```python
from build123d import *

# Parameters (mm, degrees)
BOSS_EXTRUDE1_DEPTH       = 9
SKETCH2_W                 = 3
SKETCH2_H                 = 1
SKETCH2_H_2               = 7.797958972
CUT_EXTRUDE1_DEPTH        = 19
SKETCH3_R                 = 4.5
BOSS_EXTRUDE2_DEPTH       = 6
SKETCH4_R                 = 3
BOSS_EXTRUDE3_DEPTH       = 3
F_3_0MM_DOWEL_HOLE1_D     = 3
F_3_0MM_DOWEL_HOLE1_DEPTH = 4
F_3_0MM_DOWEL_HOLE1_TIP   = 0.901290929
CUT_EXTRUDE2_DEPTH        = 3


with BuildPart() as part:
    # Sketch1 → Boss-Extrude1 (new body)
    with BuildSketch(Plane.XY):
        with BuildLine():
            ThreePointArc((-5, -4.898979486), (0, -7), (5, -4.898979486))
            Line((5, -4.898979486), (5, 4.898979486))
            ThreePointArc((5, 4.898979486), (0, 7), (-5, 4.898979486))
            Line((-5, 4.898979486), (-5, -4.898979486))
        make_face()
    extrude(amount=BOSS_EXTRUDE1_DEPTH)

    # Sketch2 → Cut-Extrude1 (cut)
    with BuildSketch(Plane.ZY.offset(5)):
        with Locations((4.5, 6.5)):
            Rectangle(SKETCH2_W, SKETCH2_H)
        with Locations((4.5, 0)):
            Rectangle(SKETCH2_W, SKETCH2_H_2)
        Polygon((3, -7), (3.352176654, -7), (6, -7), (6, -6), (3, -6), align=None)
    extrude(amount=-CUT_EXTRUDE1_DEPTH, mode=Mode.SUBTRACT)

    # Sketch3 → Boss-Extrude2 (add)
    with BuildSketch(Plane.XY.offset(9)):
        Circle(SKETCH3_R)
    extrude(amount=BOSS_EXTRUDE2_DEPTH)

    # Sketch4 → Boss-Extrude3 (add)
    with BuildSketch(Plane.XY.offset(15)):
        Circle(SKETCH4_R)
    extrude(amount=BOSS_EXTRUDE3_DEPTH)

    # Ø3.0mm Dowel Hole1
    with Locations(Plane.XY.offset(18)):
        with Locations((0, 0)):
            Hole(F_3_0MM_DOWEL_HOLE1_D / 2, depth=F_3_0MM_DOWEL_HOLE1_DEPTH)
            with Locations((0, 0, -(F_3_0MM_DOWEL_HOLE1_DEPTH + F_3_0MM_DOWEL_HOLE1_TIP / 2))):  # 118° drill point
                Cone(0, F_3_0MM_DOWEL_HOLE1_D / 2, F_3_0MM_DOWEL_HOLE1_TIP, mode=Mode.SUBTRACT)

    # Sketch9 → Cut-Extrude2 (cut)
    with BuildSketch(Plane.XY.offset(15)):
        with BuildLine():
            Line((0, 4.5), (0, 3))
            ThreePointArc((0, 3), (3, 0), (0, -3))
            Line((0, -3), (0, -4.5))
            ThreePointArc((0, -4.5), (4.5, 0), (0, 4.5))
        make_face()
    extrude(amount=-CUT_EXTRUDE2_DEPTH, mode=Mode.SUBTRACT)


solid = part.part
```
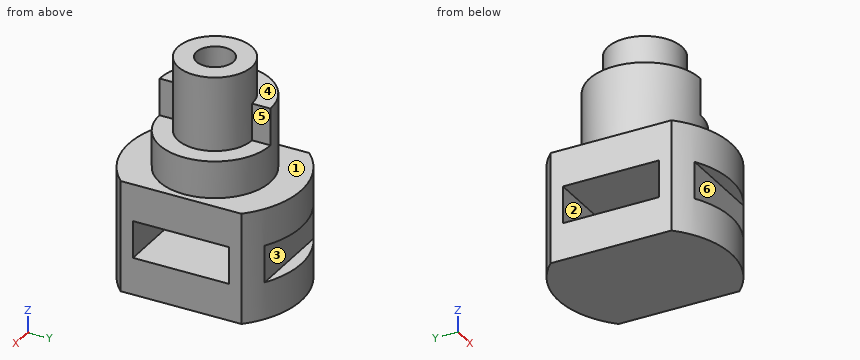
Geometry: final body of the model. Coordinates: model frame, mm. Face numbers are marked on the shaded views. A direction names the side the tool comes from. Give positions to 0.01 mm unless a question says otherwise; leave off trailing zeros. Write each loop counter-clockwise with the first axis right and the second up, starting at its lowest first coordinate (ties: lowest second). Pieces come first, ordered by that corner, then holes.
1. Section query B-B, the plane x = -2. Return loops of the section in (y, z).
2. Section query A-A, the plane z = 16.75. Return loops of the section in (x, y), then the cut area to 3 significant figures.
3. Reachability of the marked faces 1, 2 and 3 from +Z, -Z, +X, -X, +Y, -Y: full face, straight path, thin tool, end or side. Return the list, or none.
4. Draft query along Z for the marked faces 4, 5 and 6. Return one class per face: released by +Z, released by -Z, zero draft, split by the parting line, or undercut.
5. Pin query (flat end, axial travel): P1, Ø2.5, axis at x = 1, z = 4, coming from the -Y side; P2, Ø2.5, axis at x = 1, z = 4, coming from the +Y side; P3, Ø1.5, axis at x = -1.5, z = 5, coming from the -Y side. Return the tip coordinate at first contact, or that it passes through.
6. Section query D-D, the plane x = 2.5. Return loops of the section in (y, z), then the cut area to 3 significant figures.
7. Line query: probe 1 along Y at (x, z) = (0, 17.1); probe 2 along Z at (x, y) = (-3, 0.75); probe 3 along Z at (x, y) = (2.25, 6.5). Output: solid intervals per line, ascending.
8. Section query C-C, the plane z = 14.5. Return loops of the section in (x, y), then the cut area to 3 significant figures.
Computed:
1. outline: (-6.71, 0) - (6.71, 0) - (6.71, 3) - (6, 3) - (6, 6) - (6.71, 6) - (6.71, 9) - (4.03, 9) - (4.03, 15) - (2.24, 15) - (2.24, 18) - (-2.24, 18) - (-2.24, 15) - (-4.03, 15) - (-4.03, 9) - (-6.71, 9) - (-6.71, 6) - (-6, 6) - (-6, 3) - (-6.71, 3) - close; hole (-3.9, 3) - (3.9, 3) - (3.9, 6) - (-3.9, 6) - close
2. outline: circle Ø6 at (0, 0); hole circle Ø3 at (0, 0)
2. area: 21.2 mm2
3. face 1: +Z
3. face 2: +X, -X
3. face 3: +X, -X, +Y
4. face 4: released by +Z
4. face 5: zero draft
4. face 6: undercut
5. P1: stops at y = -7
5. P2: stops at y = 7
5. P3: stops at y = -6
6. outline: (-6.54, 0) - (6.54, 0) - (6.54, 3) - (6, 3) - (6, 6) - (6.54, 6) - (6.54, 9) - (3.74, 9) - (3.74, 12) - (1.66, 12) - (1.66, 18) - (-1.66, 18) - (-1.66, 12) - (-3.74, 12) - (-3.74, 9) - (-6.54, 9) - (-6.54, 6) - (-6, 6) - (-6, 3) - (-6.54, 3) - close; hole (-3.9, 3) - (3.9, 3) - (3.9, 6) - (-3.9, 6) - close
6. area: 133 mm2
7. probe 1: y = -3 to -1.5, 1.5 to 3
7. probe 2: z = 0 to 3, 6 to 15
7. probe 3: z = 0 to 3, 6 to 9
8. outline: (0, -4.5) - (0, -3) arc R3 ccw to (0, 3) - (0, 4.5) arc R4.5 ccw to start; hole circle Ø3 at (0, 0)
8. area: 38.9 mm2
